Geometry: see drawing. Coordinates: mm, zero at the bounding-box minimum. A direction names the side the tool comes from. Give positions to 0.01 mm unless a question says otherwise; leave off trailing zeros. Order: outer loops, then holes, each group sorted by start corner. A loop starts at its lowest first (then second) coordinate and runs counter-clockwise, first axis right, second up. Notation, with made-up numbers: (-15, 64.5) - (4, 64.5) arc R33 cw to (4, 95.5) - close; hole circle Ø8 at (42, 76). An arc over 180 degrees is marked (long way). Put each result on its own line as item: value. Start each with the question number.
1. Set-up query: the marked faces 5 and 6. Return all of +Z, -Z, +X, -X, +Y, -Y with unobstructed straight access to the full face (end or side cutting, diameter ignored); none if empty.
2. Ray query, line 1 along Y through (x, z) = (17.5, 44.5); line 2 along Y through (x, z) = (71.5, 36.5); line 3 along Z through (x, y) = (21, 45.5). Return the intervals inside material, ascending. Write a range as from..to.
3. Section A-A on x = 42. Return the cut outline in (y, z), plus the area to 3 significant figures.
4. Mould query, pull axis Y, two halves, no side actions, for the marked faces 1, 2, 3 and 4. Classes: pulls with the +Y half, pulls with the -Y half, needs draft (parallel to the pull), parting line crosses it, or undercut.
5. Section C-C on x = 8. Return the cut outline in (y, z), plus the area to 3 significant figures.
6. First-contact query: P1, Ø2, axis at x = 94, y = 43, coming from the -Z side. Flat tip, straight axial feed; report the tip coordinate or a pass-through.
7. Section B-B on z = 9. Return the cut outline in (x, y), plus the area to 3 significant figures.
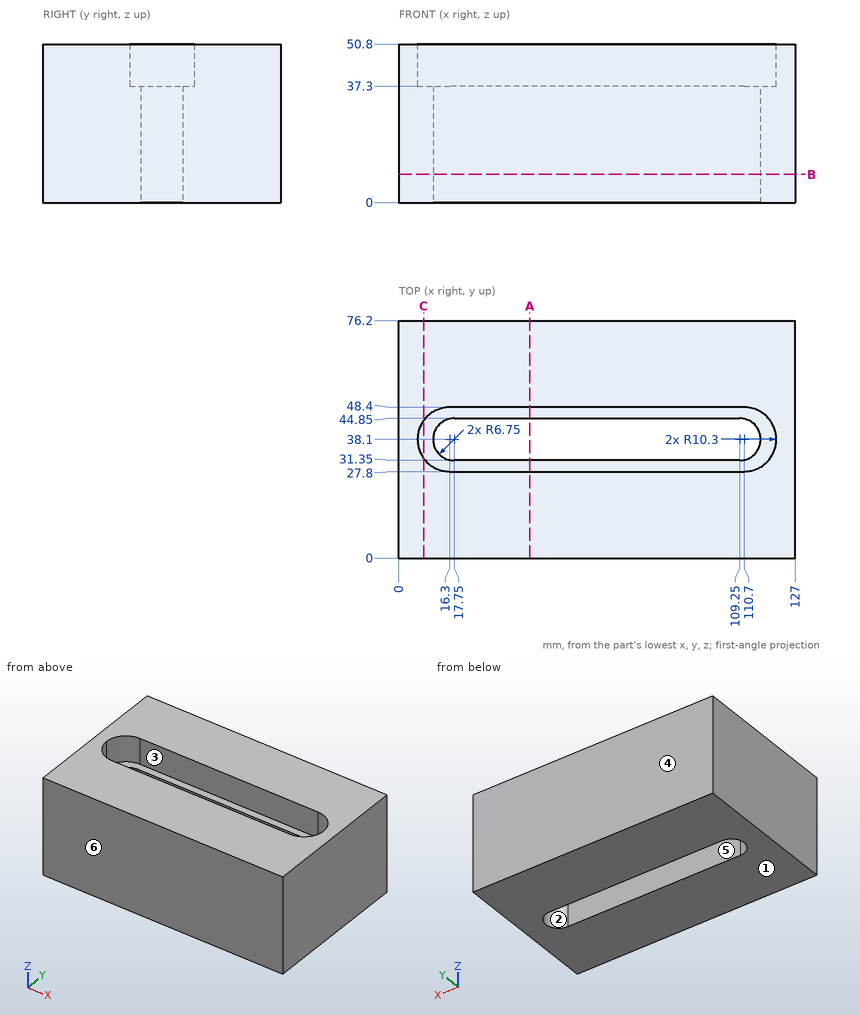
Resolved:
1. face 5: +Z, -Z
1. face 6: +Z, -Z, +X, -X, -Y
2. line 1: 0..27.8, 48.4..76.2
2. line 2: 0..31.35, 44.85..76.2
2. line 3: 0..37.3
3. outline: (0, 0) - (31.35, 0) - (31.35, 37.3) - (27.8, 37.3) - (27.8, 50.8) - (0, 50.8) - close; (44.85, 0) - (76.2, 0) - (76.2, 50.8) - (48.4, 50.8) - (48.4, 37.3) - (44.85, 37.3) - close
3. area: 3,090 mm^2
4. face 1: needs draft
4. face 2: undercut
4. face 3: undercut
4. face 4: pulls with the +Y half
5. outline: (0, 0) - (76.2, 0) - (76.2, 50.8) - (44.2, 50.8) - (44.2, 37.3) - (32, 37.3) - (32, 50.8) - (0, 50.8) - close
5. area: 3,710 mm^2
6. P1: through
7. outline: (0, 0) - (127, 0) - (127, 76.2) - (0, 76.2) - close; hole (17.75, 31.35) - (109.25, 31.35) arc R6.75 ccw to (109.25, 44.85) - (17.75, 44.85) arc R6.75 ccw to start
7. area: 8,300 mm^2
